Verification items for the finished model (mm, model axes). A direction names the side the tool comes from. Give positions to 0.01 mm unless a question says otherwise; leave off trailing zeros. Write each loop counter-clockwise with the first axis right and the second up, starting at its lowest first coordinate (ties: lowest second). Pieces come first, ordered by that corner, then holes. Notation, with made-up numbers: (85, 82.25) - (95, 82.25) arc R20 ccw to (95, 109.25) - close; hole circle Ø4 at (25, 11). An arc over 180 degrees is marked (long way). Put each result on its own line as item: value.
from build123d import *

# Parameters (mm, degrees)
BOSS_EXTRUDE1_DEPTH              = 3.175
SKETCH7_W                        = 3.175
SKETCH7_H                        = 19.05
CUT_EXTRUDE1_DEPTH               = 3.175
F_10_0_1935_DIAMETER_HOLE1_D     = 4.9149
F_10_0_1935_DIAMETER_HOLE1_DEPTH = 9.699415072
F_10_0_1935_DIAMETER_HOLE1_TIP   = 1.476584928
FILLET1_R                        = 6.35


with BuildPart() as part:
    # Sketch1 → Boss-Extrude1 (new body)
    with BuildSketch(Plane(origin=(0, 0, 0), x_dir=(0, 0, -1), z_dir=(1, 0, 0))):
        with BuildLine():
            Line((-31.934860292, 17.215678835), (23.310139708, 17.215678835))
            Line((23.310139708, 17.215678835), (23.310139708, -8.184321165))
            Line((23.310139708, -8.184321165), (0.193463217, -8.184321165))
            ThreePointArc((0.193463217, -8.184321165), (-4.215993747, -8.974380389), (-8.076831475, -11.24625986))
            Line((-8.076831475, -11.24625986), (-15.545168525, -17.65474247))
            ThreePointArc((-15.545168525, -17.65474247), (-19.406006253, -19.926621941), (-23.815463217, -20.716681165))
            Line((-23.815463217, -20.716681165), (-31.934860292, -20.716681165))
            Line((-31.934860292, -20.716681165), (-31.934860292, 17.215678835))
        make_face()
    extrude(amount=BOSS_EXTRUDE1_DEPTH)

    # Sketch7 → Cut-Extrude1 (cut)
    with BuildSketch(Plane.ZY):
        with Locations((-12.7635, 4.515678835)):
            Rectangle(SKETCH7_W, SKETCH7_H)
        with Locations((12.7635, 1.340678835)):
            Rectangle(SKETCH7_W, SKETCH7_H)
    extrude(amount=-CUT_EXTRUDE1_DEPTH, mode=Mode.SUBTRACT)

    # #10 (0.1935) Diameter Hole1
    with Locations(Plane.ZY):
        with Locations((25.4, 7.690678835), (25.4, -11.191681165), (0, 4.515678835)):
            Hole(F_10_0_1935_DIAMETER_HOLE1_D / 2, depth=F_10_0_1935_DIAMETER_HOLE1_DEPTH)
            with Locations((0, 0, -(F_10_0_1935_DIAMETER_HOLE1_DEPTH + F_10_0_1935_DIAMETER_HOLE1_TIP / 2))):  # 118° drill point
                Cone(0, F_10_0_1935_DIAMETER_HOLE1_D / 2, F_10_0_1935_DIAMETER_HOLE1_TIP, mode=Mode.SUBTRACT)

    # Fillet1
    fillet1_edges = [part.edges().sort_by_distance(p)[0] for p in [
        (1.5875, 17.215678835, 31.934860292),
        (1.5875, 17.215678835, -23.310139708),
        (1.5875, -8.184321165, -23.310139708),
        (1.5875, -20.716681165, 31.934860292),
    ]]
    fillet(fillet1_edges, radius=FILLET1_R)


solid = part.part
Q1. Go/stop test with a flat-tipped pin: pin 1 Ø1 at (x, z) = (1, 13.5) entering from -Y. Record where the tip stops, or that it passes through.
Answers follow:
pin 1: stops at y = -16.33
Q2. Section check A-A, the plane x = 1.2. Record the cut outline in (y, z).
Answers follow:
outline: (-20.72, 23.82) arc R12.7 ccw to (-17.65, 15.55) - (-11.25, 8.08) arc R12.7 cw to (-8.18, -0.19) - (-8.18, -16.96) arc R6.35 ccw to (-1.83, -23.31) - (10.87, -23.31) arc R6.35 ccw to (17.22, -16.96) - (17.22, 25.58) arc R6.35 ccw to (10.87, 31.93) - (-14.37, 31.93) arc R6.35 ccw to (-20.72, 25.58) - close; hole circle Ø4.91 at (-11.19, 25.4); hole (-8.18, 11.18) - (10.87, 11.18) - (10.87, 14.35) - (-8.18, 14.35) - close; hole (-5.01, -14.35) - (14.04, -14.35) - (14.04, -11.18) - (-5.01, -11.18) - close; hole circle Ø4.91 at (4.52, 0); hole circle Ø4.91 at (7.69, 25.4)
Q3. Release check for a two-part mould opening along Z. For faces 3 (the face through (2, -5.009, -13)), 4 (the face through (1.61, -18.81, 30.12)), 5 (the face through (2, -20.717, 25)) record: released by +Z, released by -Z, zero draft, split by the parting line, or undercut.
Answers follow:
face 3: undercut
face 4: released by +Z
face 5: zero draft
Q4. Scan lines: line 1 along Y through (x, z) = (1.65, 25.4); line 2 along Z through (x, y) = (1.5, 1.5); line 3 along Z through (x, y) = (1.3, 4.5). Record each from-to range of solid material in increasing order.
Answers follow:
line 1: y = -20.72 to -13.65, -8.73 to 5.23, 10.15 to 17.22
line 2: z = -23.31 to -14.35, -11.18 to 11.18, 14.35 to 31.93
line 3: z = -23.31 to -14.35, -11.18 to -2.46, 2.46 to 11.18, 14.35 to 31.93
Q5. Section check B-B, the plane z = -8.5. Record the cut outline in (x, y) (3 decimals).
Answers follow:
outline: (0, -8.184) - (3.175, -8.184) - (3.175, 17.216) - (0, 17.216) - close
Q6. Set-up check for faces 1 (the face through (2, 14.041, -13)), 2 (the face through (1.61, 15.4, 30.03)): record each of +Z, -Z, +X, -X, +Y, -Y from which the full face is reachable in a straight line by a thin tool's end or side.
Answers follow:
face 1: +X, -X
face 2: +Z, +X, -X, +Y
